Work out the finished part from the listing and answer in its coordinate system (mm). Coordinates: 2 decimals unless noted, no trailing zeros. Order: outer loops, then holes, each group sorted by start corner. A loop starts at its lowest first (then second) coordinate and runs counter-clockwise, first axis right, second up. Notation, with made-up numbers: (-21.75, -4.75) -> (1.25, -4.75) arc R18 ccw to (1.25, 14.25) -> close; hole circle Ø11 at (6.25, 69.5). An arc over 180 degrees is marked (long way). Write item = value, one per line. Start each with the question number.
Q1. The part is cut by section C-C, the plane z = 4.6. Determine the outline of the cut face in (x, y), plus the area to 3 significant figures.
Q2. For a pull along X with two mould halves and no side action, classify faces 1 (the cylindrical face through (14.43, 10.4, 2.79)), 2 (the cylindrical face through (-14.43, -10.4, 2.79)), 3 (the cylindrical face through (11.4, 8.8, 2.8)), 4 (the cylindrical face through (11.4, -7.2, 2.8)) as +X half, -X half, draft (parallel to the pull), parting line (faces both ways), or undercut.
Q3. The part is cut by section A-A, the plane y = 8. Determine the outline of the cut face in (x, z).
Q4. Straight lines are drawn through the part: L1, parallel to Y at x = 12, z = 4.45; L2, parallel to X at y = -8, z = 3.3; L3, parallel to X at y = 8.75, z = 0.55. For each, find the intervals that lie inside material, in ascending order. Write a range as from..to.
Q5. A flat-ended cylindrical pin translates along its axis: pin 1 (1.2 mm diameter, centred on x = -12, y = -8, fed in from +Z). Find the tip coordinate at first contact, or state that the pin passes through.
Q6. The part is cut by section B-B, the plane x = -12. Determine the outline of the cut face in (y, z).
Solid Edge part; units mm, degrees
sketch "Sketch1" plane through (0, 0, 0) normal (0, 0, 1) x (1, 0, 0)
  line L0 (15, -11) -> (-15, -11)
  line L1 (-15, -11) -> (-15, 11)
  line L2 (-15, 11) -> (15, 11)
  line L3 (15, 11) -> (15, -11)
  dimension "D1" = 15
  dimension "D2" = 15
extrude "Protrusion1" add sketch "Sketch1" along normal blind 5.5
hole "Hole_1" at (12, 8, 5.5) direction (0, 0, -1) diameter 2 end through all
hole "Hole1" at (12, -8, 5.5) direction (0, 0, -1) diameter 2 end through all
hole "Hole2" at (-12, 8, 5.5) direction (0, 0, -1) diameter 2 end through all
hole "Hole3" at (-12, -8, 5.5) direction (0, 0, -1) diameter 2 end through all
fillet "Round_1" radius 2 3 edges at (-15, 11, 2.75) (-15, -11, 2.75) (15, -11, 2.75)
fillet "Round_2" radius 2 1 edges at (15, 11, 2.75)
properties material "木材, アッシュ"
Model answer:
q1.outline = (-15, -9) arc R2 ccw to (-13, -11) -> (13, -11) arc R2 ccw to (15, -9) -> (15, 9) arc R2 ccw to (13, 11) -> (-13, 11) arc R2 ccw to (-15, 9) -> close; hole circle Ø2 at (-12, -8); hole circle Ø2 at (-12, 8); hole circle Ø2 at (12, -8); hole circle Ø2 at (12, 8)
q1.area = 644 mm2
q2.face_1 = +X half
q2.face_2 = -X half
q2.face_3 = undercut
q2.face_4 = undercut
q3.outline = (-15, 0) -> (-13, 0) -> (-13, 5.5) -> (-15, 5.5) -> close; (-11, 0) -> (11, 0) -> (11, 5.5) -> (-11, 5.5) -> close; (13, 0) -> (15, 0) -> (15, 5.5) -> (13, 5.5) -> close
q4.L1 = -11..-9, -7..7, 9..11
q4.L2 = -15..-13, -11..11, 13..15
q4.L3 = -15..-12.66, -11.34..11.34, 12.66..15
q5.pin_1 = through
q6.outline = (-11, 0) -> (-9, 0) -> (-9, 5.5) -> (-11, 5.5) -> close; (-7, 0) -> (7, 0) -> (7, 5.5) -> (-7, 5.5) -> close; (9, 0) -> (11, 0) -> (11, 5.5) -> (9, 5.5) -> close
